```python
from build123d import *

# Parameters (mm, degrees)
RESSALTO_EXTRUS_O1_DEPTH = 2
ESBO_O2_R                = 0.995647449
CORTE_EXTRUS_O1_DEPTH    = 2


with BuildPart() as part:
    # Esboço1 → Ressalto-extrusão1 (new body)
    with BuildSketch(Plane(origin=(0, 0, 0), x_dir=(1, 0, 0), z_dir=(0, 1, 0))):
        with BuildLine():
            Line((-0.5, 35.495613698), (-0.5, 28.495613698))
            ThreePointArc((-0.5, 28.495613698), (0, -28.5), (0.5, 28.495613698))
            Line((0.5, 28.495613698), (0.5, 35.495613698))
            ThreePointArc((0.5, 35.495613698), (2.33575042, 35.209276303), (3.8486175, 34.130757919))
            ThreePointArc((3.8486175, 34.130757919), (5.24059873, 32.366531639), (7.168579512, 31.211977086))
            ThreePointArc((7.168579512, 31.211977086), (0, -34), (-7.168579512, 31.211977086))
            ThreePointArc((-7.168579512, 31.211977086), (-5.24059873, 32.366531639), (-3.8486175, 34.130757919))
            ThreePointArc((-3.8486175, 34.130757919), (-2.33575042, 35.209276303), (-0.5, 35.495613698))
        make_face()
    extrude(amount=RESSALTO_EXTRUS_O1_DEPTH)

    # Esboço2 → Corte-extrusão1 (cut)
    with BuildSketch(Plane(origin=(0, 2, 0), x_dir=(1, 0, 0), z_dir=(0, 1, 0))):
        with Locations(Location((-2.373103124, 32.484243676, 0), (0, 0, 270))):
            Circle(ESBO_O2_R)
        with Locations(Location((2.373103124, 32.484243676, 0), (0, 0, 90))):
            Circle(ESBO_O2_R)
    extrude(amount=-CORTE_EXTRUS_O1_DEPTH, mode=Mode.SUBTRACT)


solid = part.part
```
Geometry: final body of the model. Coordinates: model frame, mm. A direction names the side the tool comes from. Round coordinates to 2 decimals unless told otherwise and drop trailing zeros. Order: outer loops, then holes, each group sorted by start corner. A loop starts at its lowest first (then second) coordinate and runs counter-clockwise, first axis right, second up. Notation, with made-up numbers: (19, 8) -> (43, 8) arc R13 ccw to (43, 27) -> close; hole circle Ø1 at (-36.5, 28). An arc over 180 degrees is marked (long way). Use one line per item in the form item = value. Start each with the question number.
1. Reachability of faces 1 (the face through (-5.26, 0.99, -32.35)), 2 (the face through (-0.5, 1, -32)) from +Z, -Z, +X, -X, +Y, -Y: full face, straight path, thin tool, end or side. Return the list, or none.
2. Draft query along Z for faces 3 (the face through (0.5, 1, -32)), 4 (the face through (-2.33, 1.01, -33.48)), 5 (the face through (-2.36, 0.99, -35.2)). Return one class per face: pulls with the +Z half, pulls with the -Z half, needs draft (parallel to the pull), parting line crosses it, or undercut.
3. Pin query (flat end, axial travel): pin 1 Ø0.6 at (y, z) = (1, -33.5) entering from -X; pin 2 Ø1.8 at (x, z) = (2.37, -32.48) entering from +Y. Return the tip coordinate at first contact, or that it passes through.
4. Cut plane B-B (x = -24). Return the cut outline in (y, z), then the cut area to 3 significant figures.
5. Cut plane C-C (y = 1). Return the cut outline in (x, z).
6. Line query: probe 1 along X at (y, z) = (0.75, 0); probe 2 along X at (y, z) = (1.1, 23); probe 3 along Z at (x, y) = (17.5, 0.6). Output: solid intervals per line, ascending.
7. Cut plane A-A (z = 1). Return the cut outline in (x, y), then the cut area to 3 significant figures.
Solution:
q1.face_1 = -Z, -X, +Y, -Y
q1.face_2 = -Z, +Y, -Y
q2.face_3 = needs draft
q2.face_4 = undercut
q2.face_5 = pulls with the -Z half
q3.pin_1 = -4.45
q3.pin_2 = through
q4.outline = (0, -21.65) -> (2, -21.65) -> (2, -15.37) -> (0, -15.37) -> close; (0, 15.37) -> (2, 15.37) -> (2, 23.65) -> (0, 23.65) -> close
q4.area = 29.1 mm^2
q5.outline = (-7.17, -31.21) arc R6.22 cw to (-3.85, -34.13) arc R4.04 ccw to (-0.5, -35.5) -> (-0.5, -28.5) arc R28.5 cw (long way) to (0.5, -28.5) -> (0.5, -35.5) arc R4.04 ccw to (3.85, -34.13) arc R6.22 cw to (7.17, -31.21) arc R33 ccw (long way) to start; hole circle Ø1.99 at (-2.37, -32.48); hole circle Ø1.99 at (2.37, -32.48)
q6.probe_1 = -32.98 to -28.5, 28.5 to 32.98
q6.probe_2 = -24.6 to -16.83, 16.83 to 24.6
q6.probe_3 = -26.98 to -22.49, 22.49 to 28.98
q7.outline = (-33, 0) -> (-28.48, 0) -> (-28.48, 2) -> (-33, 2) -> close; (28.48, 0) -> (33, 0) -> (33, 2) -> (28.48, 2) -> close
q7.area = 18.1 mm^2
